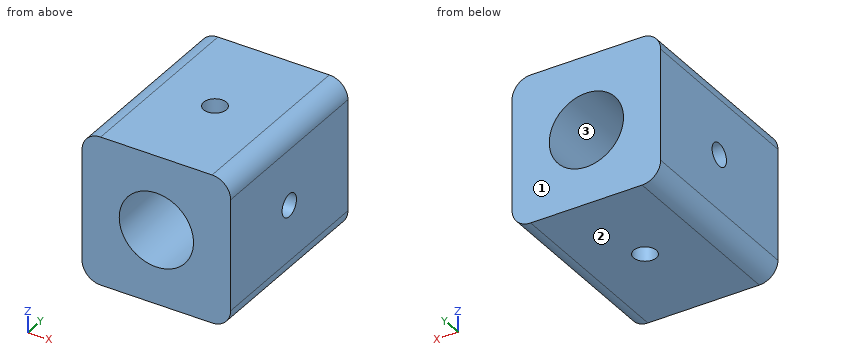
Autodesk Inventor part; units mm, degrees
ref_plane "YZ Plane" through (0, 0, 0) normal (1, 0, 0) x (0, 1, 0)
ref_plane "XZ Plane" through (0, 0, 0) normal (0, 1, 0) x (-1, 0, 0)
ref_plane "XY Plane" through (0, 0, 0) normal (0, 0, 1) x (1, 0, 0)
sketch "Sketch1" plane through (0, 0, 0) normal (0, 1, 0) x (-1, 0, 0)
  circle A0 centre (0, 0) radius 4
  line L0 (6, 8) -> (-6, 8)
  line L1 (-8, 6) -> (-8, -6)
  line L2 (-6, -8) -> (6, -8)
  line L3 (8, -6) -> (8, 6)
  line L4 (8, 8) -> (-8, -8) construction
  line L5 (-8, 8) -> (8, -8) construction
  arc A1 (8, 6) -> (6, 8) centre (6, 6) ccw
  arc A2 (6, -8) -> (8, -6) centre (6, -6) ccw
  arc A3 (-8, -6) -> (-6, -8) centre (-6, -6) ccw
  arc A4 (-6, 8) -> (-8, 6) centre (-6, 6) ccw
  dimension "d0" = 8
  dimension "d1" = 16
  dimension "d2" = 16
  dimension "d5" = 2
extrude "Extrusion1" add sketch "Sketch1" along normal blind 20
sketch "Sketch2" plane through (-6, 0, 8) normal (0, 0, 1) x (1, 0, 0)
  line L0 (0, 0) -> (12, 0)
  line L1 (12, 0) -> (12, 20)
  line L2 (0, 20) -> (12, 20)
  line L3 (0, 0) -> (0, 20)
  point P0 (6, 0)
  point P1 (6, 10)
  dimension "d6" = 6
hole "Hole1" at (0, 10, 8) direction (0, 0, -1) diameter 2.45 depth 3 tip angle 118
pattern_circular "Circular Pattern1" count 4 over 360 about axis through (0, -10, 0) along (0, 1, 0) of "Hole1"
thread "Thread1"
properties part number "leadscrew"
Geometry check sheet. Reference: the model listing, model coordinates, mm. Face numbers are marked on the shaded views. Coordinates: 2 decimals unless noted, no trailing zeros. Order: outer loops, then holes, each group sorted by start corner. A loop starts at its lowest first (then second) coordinate and runs counter-clockwise, first axis right, second up. Notation, with made-up numbers: (41, 4.5) - (63, 4.5) arc R18 ccw to (63, 22.5) - close; hole circle Ø4 at (27, 7.5). An arc over 180 degrees is marked (long way). Answer in a Markdown table with one row per item. Add a question column.
1) Cross-section at B-B, the plane z = -1.75. Record the cut outline in (x, y), then the cut area to 3 significant figures.
2) Release check for a two-part mould opening along Z. For the marked faces 1, 2 and 3 record: +Z half, -Z half, draft (parallel to the pull), parting line (faces both ways), or undercut.
3) Material ranges on line 1 along X through (y, z) = (10, -5.5) (3 decimals); line 2 along Z through (x, y) = (0, 15.75); line 3 along Y through (x, z) = (0, 5.85) (3 decimals), recorded low to high. Write a range as [from, to].
4) Cross-section at A-A, the plane y = 13. Record the cut outline in (x, z), then the cut area to 3 significant figures.
5) Cross-section at C-C, the plane x = -2.25. Record the cut outline in (y, z), then the cut area to 3 significant figures.
6) Gauge pin test, flat ends, axial feed: P1, Ø1.5, axis at y = 10, z = 0, coming from the +X side; P2, Ø3, axis at x = 0, y = 10, coming from the +Z side. Record the tip position at first contact, or that the pin passes through.
Check result:
| question | item | result |
|---|---|---|
| 1 | outline | (-8, 0) - (-3.6, 0) - (-3.6, 20) - (-8, 20) - close; (3.6, 0) - (8, 0) - (8, 20) - (3.6, 20) - close |
| 1 | area | 176 mm² |
| 2 | face 1 | draft |
| 2 | face 2 | -Z half |
| 2 | face 3 | undercut |
| 3 | line 1 | x = [-8, -1.225], [1.225, 8] |
| 3 | line 2 | z = [-8, -4], [4, 8] |
| 3 | line 3 | y = [0, 8.775], [11.225, 20] |
| 4 | outline | (-8, -6) arc R2 ccw to (-6, -8) - (6, -8) arc R2 ccw to (8, -6) - (8, 6) arc R2 ccw to (6, 8) - (-6, 8) arc R2 ccw to (-8, 6) - close; hole circle Ø8 at (0, 0) |
| 4 | area | 202 mm² |
| 5 | outline | (0, -8) - (20, -8) - (20, -3.31) - (0, -3.31) - close; (0, 3.31) - (20, 3.31) - (20, 8) - (0, 8) - close |
| 5 | area | 188 mm² |
| 6 | P1 | stops at x = 4.71 |
| 6 | P2 | stops at z = 8 |
